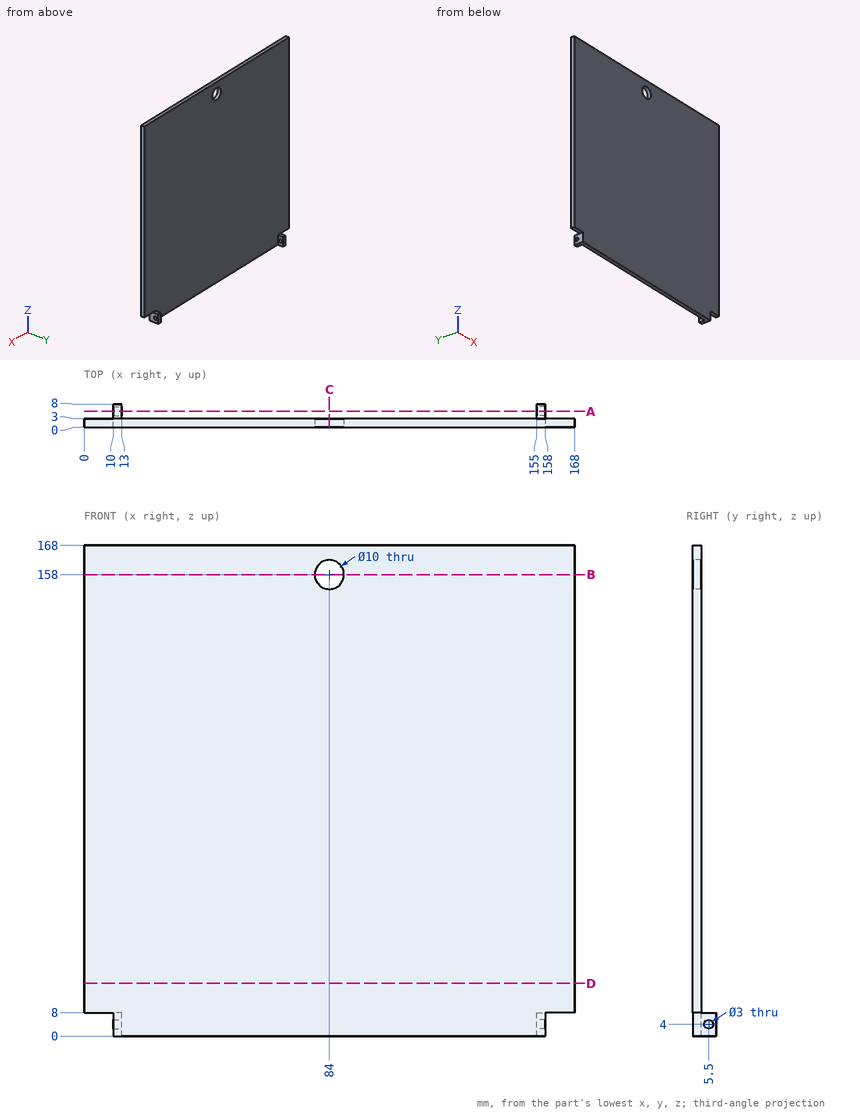
Print and shaded views of the part. All mm, measured from the part's lowest x, y and z. Coordinates: 2 decimals unless noted, no trailing zeros. Loops run counter-clockwise (first coordinate to the right, second up) from the corner with the lowest first, then second, coordinate; pieces in that order, holes last. Notation, with made-up numbers: M 12.5,-36 L 39.5,-36 A6 cw 39.5,-30 Z; hole C 3,-31 d4. An arc over 180 degrees is marked long. Use a Markdown table: item, result. Add a question column.
Q1. Pin check, flat tips, straight feed: P1, Ø1.5, axis at y = 5, z = 2, coming from the -X side; P2, Ø6, axis at x = 84, z = 158, coming from the -Y side; P3, Ø0.9, axis at x = 11, y = 5.5, coming from the +Z side; P4, Ø2.5, axis at x = 163, y = 1.5, coming from the -Z side. Stop position of each tip, or through.
Q2. Cut at D-D (z = 18). Write the cut outline in (x, y).
Q3. Cut at A-A (y = 5.5). Write the cut outline in (x, z).
Q4. Probe L1, parallel to Z at x = 156.2, y = 5.5; L2, parallel to Y at x = 11.6, z = 4; L3, parallel to X at y = 1.5, z = 158. List the from-to ranges inside material, lowest first.
Q5. Cut at C-C (x = 84). Write the cut outline in (y, z), and give its area (3 significant figures).
Q6. Cut at B-B (z = 158). Write the cut outline in (x, y), and give its area (3 significant figures).
Worked out:
| question | item | result |
|---|---|---|
| 1 | P1 | stops at x = 10 |
| 1 | P2 | passes through |
| 1 | P3 | stops at z = 8 |
| 1 | P4 | stops at z = 8 |
| 2 | outline | M 0,0 L 168,0 L 168,3 L 0,3 Z |
| 3 | outline | M 10,0 L 13,0 L 13,2.5 L 10,2.5 Z; M 10,5.5 L 13,5.5 L 13,8 L 10,8 Z; M 155,0 L 158,0 L 158,2.5 L 155,2.5 Z; M 155,5.5 L 158,5.5 L 158,8 L 155,8 Z |
| 4 | L1 | z = 0 to 2.5, 5.5 to 8 |
| 4 | L2 | y = 0 to 4, 7 to 8 |
| 4 | L3 | x = 0 to 79, 89 to 168 |
| 5 | outline | M 0,0 L 3,0 L 3,153 L 0,153 Z; M 0,163 L 3,163 L 3,168 L 0,168 Z |
| 5 | area | 474 mm2 |
| 6 | outline | M 0,0 L 79,0 L 79,3 L 0,3 Z; M 89,0 L 168,0 L 168,3 L 89,3 Z |
| 6 | area | 474 mm2 |
